Verification items for the finished model (mm, model axes). Face numbers are marked on the shaded views. A direction names the side the tool comes from. Round coordinates to 2 decimals unless told otherwise and drop trailing zeros. Order: outer loops, then holes, each group sorted by start corner. A loop starts at its lowest first (then second) coordinate and runs counter-clockwise, first axis right, second up. Notation, with made-up numbers: M 49.5,-25 L 57.5,-25 A25 ccw 57.5,11 Z; hole C 17.25,82.25 d8. An arc over 180 degrees is marked long. One line per item, written item: value. Start each with the question number.
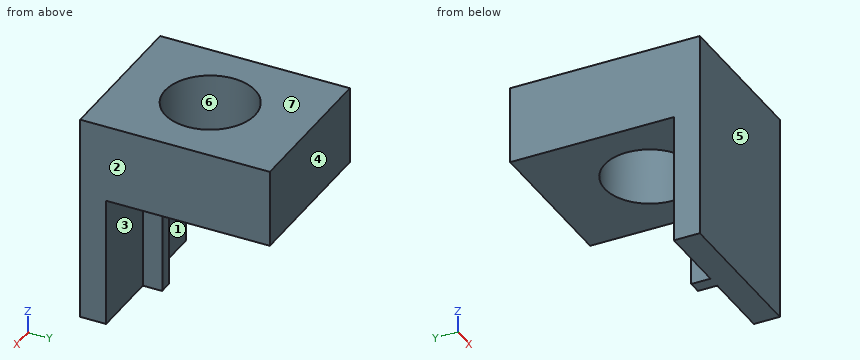
from build123d import *

# Parameters (mm, degrees)
SKETCH1_W           = 38.1
SKETCH1_H           = 50.8
BOSS_EXTRUDE1_DEPTH = 6.35
SKETCH2_W           = 3.175
SKETCH2_H           = 50.8
BOSS_EXTRUDE2_DEPTH = 6.35
SKETCH3_W           = 38.1
SKETCH3_H           = 19.05
BOSS_EXTRUDE3_DEPTH = 40
SKETCH4_R           = 11
CUT_EXTRUDE1_DEPTH  = 72.357305162


with BuildPart() as part:
    # Sketch1 → Boss-Extrude1 (new body)
    with BuildSketch(Plane(origin=(0, 0, 0), x_dir=(1, 0, 0), z_dir=(0, 1, 0))):
        Rectangle(SKETCH1_W, SKETCH1_H)
    extrude(amount=BOSS_EXTRUDE1_DEPTH)

    # Sketch2 → Boss-Extrude2 (add)
    with BuildSketch(Plane(origin=(0, 6.35, 0), x_dir=(1, 0, 0), z_dir=(0, 1, 0))):
        Rectangle(SKETCH2_W, SKETCH2_H)
    extrude(amount=BOSS_EXTRUDE2_DEPTH)

    # Sketch3 → Boss-Extrude3 (add)
    with BuildSketch(Plane(origin=(0, 6.35, 0), x_dir=(1, 0, 0), z_dir=(0, 1, 0))):
        with Locations((0, -15.875)):
            Rectangle(SKETCH3_W, SKETCH3_H)
    extrude(amount=BOSS_EXTRUDE3_DEPTH)

    # Sketch4 → Cut-Extrude1 (cut, through all)
    with BuildSketch(Plane.XY.offset(25.4)):
        with Locations((0, 22)):
            Circle(SKETCH4_R)
    extrude(amount=-CUT_EXTRUDE1_DEPTH, mode=Mode.SUBTRACT)


solid = part.part
1. Section check C-C (x = 0). Record the cut outline in (y, z).
2. Depth check by flat-ended pin: pin 1 (3 mm diameter, centred on x = -4.5, y = 13.5, fed in from -Z); pin 2 (3 mm diameter, centred on x = -15, z = -13, fed in from +Y); pin 3 (1.4 mm diameter, centred on y = 8.5, z = -17.5, fed in from -X). Enter the tip coordinate at first touch or a pass-through.
3. Section check A-A (y = 22). Record the cut outline in (x, z).
4. Section check D-D (y = 7). Record the cut outline in (x, z).
5. Scan lines: line 1 along X through (y, z) = (22, 15); line 2 along Y through (x, z) = (0, 14); line 3 along Y through (x, z) = (2, -14). Record each from-to range of solid material in increasing order.
6. Section check B-B (z = -0.5). Record the cut outline in (x, y).
7. Draft check along Y on the marked faces 4, 5, 6 and 7. Enter one of: released by +Y, released by -Y, zero draft, split by the parting line, or undercut.
8. Tool access check on the marked faces 1, 2 and 3. Record the directions out of +Z, -Z, +X, -X, +Y, -Y that give a thin tool (end or side, any length) a straight path to the whole face; none if there is none.
Geometry check:
1. outline: M 0,-25.4 L 11,-25.4 L 11,25.4 L 0,25.4 Z; M 33,6.35 L 46.35,6.35 L 46.35,25.4 L 33,25.4 Z
2. pin 1: stops at z = 6.35
2. pin 2: stops at y = 6.35
2. pin 3: stops at x = -1.59
3. outline: M -19.05,6.35 L -11,6.35 L -11,25.4 L -19.05,25.4 Z; M 11,6.35 L 19.05,6.35 L 19.05,25.4 L 11,25.4 Z
4. outline: M -19.05,6.35 L -1.59,6.35 L -1.59,-25.4 L 1.59,-25.4 L 1.59,6.35 L 19.05,6.35 L 19.05,25.4 L -19.05,25.4 Z
5. line 1: x = -19.05 to -11, 11 to 19.05
5. line 2: y = 0 to 11, 33 to 46.35
5. line 3: y = 0 to 6.35
6. outline: M -19.05,0 L 19.05,0 L 19.05,6.35 L 1.59,6.35 L 1.59,11.12 A11 cw -1.59,11.12 L -1.59,6.35 L -19.05,6.35 Z
7. face 4: released by +Y
7. face 5: released by -Y
7. face 6: undercut
7. face 7: zero draft
8. face 1: -Z, -X, +Y
8. face 2: +Z, -Z, +X, +Y, -Y
8. face 3: -Z, +X, +Y
